from build123d import *

# Parameters (mm, degrees)
F0_W     = 8.912432854
F0_H     = 0.0079375
F0_W_2   = 2.54
F0_W_3   = 18.0631426697
F1_DEPTH = 2.1082


with BuildPart() as f1:
    # F0 (on Right) → F1 (new body)
    with BuildSketch(Plane.YZ):
        with BuildLine():
            Line((0, 162.0091375), (0, 0))
            Line((0, 0), (12.335197777, 0))
            Line((12.335197777, 0), (18.8042013144, 29.896105485))
            Line((18.8042013144, 29.896105485), (30.5493542935, 2.3257501254))
            Line((30.5493542935, 2.3257501254), (31.5401391658, 0))
            Line((31.5401391658, 0), (31.5707651968, 0))
            Line((31.5707651968, 0), (40.8442968098, 0))
            Line((40.8442968098, 0), (20.5594925834, 47.616175108))
            Line((20.5594925834, 47.616175108), (39.5771112022, 135.5049402038))
            Line((39.5771112022, 135.5049402038), (73.5248959406, 160.7899383022))
            Line((73.5248959406, 160.7899383022), (100.203, 160.7899383022))
            Line((100.203, 160.7899383022), (100.203, 162.0091375))
            Line((100.203, 162.0091375), (82.1398573303, 162.0091375))
            ThreePointArc((82.1398573303, 162.0091375), (80.3438061061, 162.7530862758), (79.5998573303, 164.5491375))
            Line((79.5998573303, 164.5491375), (79.5998573303, 169.3418))
            Line((79.5998573303, 169.3418), (70.6874244764, 169.3418))
            Line((70.6874244764, 169.3418), (70.6874244764, 165.8480664454))
            Line((70.6874244764, 165.8480664454), (70.6874244764, 164.5491375))
            ThreePointArc((70.6874244764, 164.5491375), (70.0510915867, 162.8675752701), (68.4609272063, 162.0285589874))
            ThreePointArc((68.4609272063, 162.0285589874), (68.3044763435, 162.0139975214), (68.1474244764, 162.0091375))
            Line((68.1474244764, 162.0091375), (0, 162.0091375))
        make_face()
        Polygon((21.4843682503, 35.8535070154), (23.4753466245, 31.1799211209), (21.1385536773, 30.1844319338), (19.147575303, 34.8580178283), align=None, mode=Mode.SUBTRACT)
        Polygon((25.8665425285, 25.5668719827), (27.8575209028, 20.8932860882), (25.5207279555, 19.8977969011), (23.5297495813, 24.5713827956), align=None, mode=Mode.SUBTRACT)
        with BuildLine():
            Line((12.3986134924, 50.3752630702), (11.6175919588, 46.7658196656))
            Line((11.6175919588, 46.7658196656), (10.5918, 46.7658196656))
            Line((10.5918, 46.7658196656), (10.5918, 158.7579375))
            Line((10.5918, 158.7579375), (35.8507619547, 158.7579375))
            Line((35.8507619547, 158.7579375), (31.8897708968, 140.4524587956))
            Line((31.8897708968, 140.4524587956), (31.1087493632, 136.8430153909))
            Line((31.1087493632, 136.8430153909), (35.5475592049, 135.882533211))
            ThreePointArc((35.5475592049, 135.882533211), (37.1456481821, 134.7755682604), (37.4929253116, 132.8628062845))
            Line((37.4929253116, 132.8628062845), (29.5595533377, 96.1992113407))
            ThreePointArc((29.5595533377, 96.1992113407), (28.452588387, 94.6011223635), (26.5398264112, 94.2538452339))
            Line((26.5398264112, 94.2538452339), (22.1010165695, 95.2143274138))
            Line((22.1010165695, 95.2143274138), (21.7536814278, 93.6091392306))
            Line((21.7536814278, 93.6091392306), (21.4063462861, 92.0039510473))
            Line((21.4063462861, 92.0039510473), (25.8451561277, 91.0434688674))
            ThreePointArc((25.8451561277, 91.0434688674), (27.4432451049, 89.9365039168), (27.7905222345, 88.0237419409))
            Line((27.7905222345, 88.0237419409), (19.8571502605, 51.3601469971))
            ThreePointArc((19.8571502605, 51.3601469971), (18.7501853099, 49.7620580199), (16.837423334, 49.4147808903))
            Line((16.837423334, 49.4147808903), (12.3986134924, 50.3752630702))
        make_face(mode=Mode.SUBTRACT)
        Polygon((47.0613097153, 149.2568137468), (48.5785484084, 147.2197602993), (44.5044415132, 144.1852829132), (42.9872028202, 146.2223363607), align=None, mode=Mode.SUBTRACT)
        Polygon((44.8088104432, 150.074821282), (46.6876875952, 158.7579375), (56.4668125154, 158.7579375), align=None, mode=Mode.SUBTRACT)
        Polygon((63.2751536106, 161.3332132886), (64.7923923036, 159.296159841), (60.7182854085, 156.2616824549), (59.2010467154, 158.2987359025), align=None, mode=Mode.SUBTRACT)
        with BuildLine():
            Line((0, 164.5491375), (0, 162.0091375))
            Line((0, 162.0091375), (68.1474244764, 162.0091375))
            ThreePointArc((68.1474244764, 162.0091375), (68.3044763435, 162.0139975214), (68.4609272063, 162.0285589874))
            Line((68.4609272063, 162.0285589874), (69.6856973646, 162.9407926238))
            Line((69.6856973646, 162.9407926238), (68.1474244764, 165.0060867035))
            Line((68.1474244764, 165.0060867035), (68.1474244764, 164.5491375))
            Line((68.1474244764, 164.5491375), (55.1748093832, 164.5491375))
            Line((55.1748093832, 164.5491375), (50.0948093832, 164.5491375))
            Line((50.0948093832, 164.5491375), (10.3999171089, 164.5491375))
            Line((10.3999171089, 164.5491375), (5.3199171089, 164.5491375))
            Line((5.3199171089, 164.5491375), (0, 164.5491375))
        make_face()
        Polygon((18.8042013144, 29.896105485), (12.335197777, 0), (13.2072197655, 0), (31.5401391658, 0), (30.5493542935, 2.3257501254), align=None)
        Polygon((0, 169.3418), (0, 164.5491375), (5.3199171089, 164.5491375), (5.3199171089, 167.0891375), (10.3999171089, 167.0891375), (10.3999171089, 164.5491375), (50.0948093832, 164.5491375), (50.0948093832, 167.0891375), (55.1748093832, 167.0891375), (55.1748093832, 164.5491375), (68.1474244764, 164.5491375), (68.1474244764, 165.0060867035), (68.1474244764, 169.3418), align=None)
        with BuildLine():
            Line((69.6856973646, 162.9407926238), (68.4609272063, 162.0285589874))
            ThreePointArc((68.4609272063, 162.0285589874), (70.0510915867, 162.8675752701), (70.6874244764, 164.5491375))
            Line((70.6874244764, 164.5491375), (70.6874244764, 165.8480664454))
            Line((70.6874244764, 165.8480664454), (70.6874244764, 169.3418))
            Line((70.6874244764, 169.3418), (68.1474244764, 169.3418))
            Line((68.1474244764, 169.3418), (68.1474244764, 165.0060867035))
            Line((68.1474244764, 165.0060867035), (69.6856973646, 162.9407926238))
        make_face()
        with Locations((75.1436409033, 169.34576875)):
            Rectangle(F0_W, F0_H)
        with Locations((80.8698573303, 169.34576875)):
            Rectangle(F0_W_2, F0_H)
        with BuildLine():
            Line((82.1398573303, 169.3418), (79.5998573303, 169.3418))
            Line((79.5998573303, 169.3418), (79.5998573303, 164.5491375))
            ThreePointArc((79.5998573303, 164.5491375), (80.3438061061, 162.7530862758), (82.1398573303, 162.0091375))
            Line((82.1398573303, 162.0091375), (100.203, 162.0091375))
            Line((100.203, 162.0091375), (100.203, 164.5491375))
            Line((100.203, 164.5491375), (89.6502663064, 164.5491375))
            Line((89.6502663064, 164.5491375), (84.5702663064, 164.5491375))
            Line((84.5702663064, 164.5491375), (82.1398573303, 164.5491375))
            Line((82.1398573303, 164.5491375), (82.1398573303, 169.3418))
        make_face()
        with Locations((91.1714286652, 169.34576875)):
            Rectangle(F0_W_3, F0_H)
        Polygon((100.203, 169.3418), (82.1398573303, 169.3418), (82.1398573303, 164.5491375), (84.5702663064, 164.5491375), (84.5702663064, 167.0891375), (89.6502663064, 167.0891375), (89.6502663064, 164.5491375), (100.203, 164.5491375), align=None)
        Polygon((10.5918, 46.7658196656), (11.6175919588, 46.7658196656), (12.3986134924, 50.3752630702), (12.9357939022, 52.8578095868), (20.8691658762, 89.5214045307), (21.4063462861, 92.0039510473), (21.7536814278, 93.6091392306), (22.1010165695, 95.2143274138), (22.6381969794, 97.6968739305), (30.5715689534, 134.3604688743), (31.1087493632, 136.8430153909), (31.8897708968, 140.4524587956), (35.8507619547, 158.7579375), (10.5918, 158.7579375), align=None)
        with BuildLine():
            Line((12.9357939022, 52.8578095868), (12.3986134924, 50.3752630702))
            Line((12.3986134924, 50.3752630702), (16.837423334, 49.4147808903))
            ThreePointArc((16.837423334, 49.4147808903), (18.7501853099, 49.7620580199), (19.8571502605, 51.3601469971))
            Line((19.8571502605, 51.3601469971), (27.7905222345, 88.0237419409))
            ThreePointArc((27.7905222345, 88.0237419409), (27.4432451049, 89.9365039168), (25.8451561277, 91.0434688674))
            Line((25.8451561277, 91.0434688674), (21.4063462861, 92.0039510473))
            Line((21.4063462861, 92.0039510473), (20.8691658762, 89.5214045307))
            Line((20.8691658762, 89.5214045307), (25.3079757178, 88.5609223508))
            Line((25.3079757178, 88.5609223508), (24.0175885553, 82.5974767434))
            Line((24.0175885553, 82.5974767434), (22.9432277355, 77.6323837102))
            Line((22.9432277355, 77.6323837102), (19.7419229759, 62.8377489213))
            Line((19.7419229759, 62.8377489213), (18.6675621562, 57.872655888))
            Line((18.6675621562, 57.872655888), (17.3746037439, 51.8973274069))
            Line((17.3746037439, 51.8973274069), (12.9357939022, 52.8578095868))
        make_face()
        Polygon((20.8691658762, 89.5214045307), (12.9357939022, 52.8578095868), (17.3746037439, 51.8973274069), (18.6675621562, 57.872655888), (16.1850156395, 58.4098362979), (17.2593764593, 63.3749293312), (19.7419229759, 62.8377489213), (22.9432277355, 77.6323837102), (20.4606812189, 78.16956412), (21.5350420386, 83.1346571533), (24.0175885553, 82.5974767434), (25.3079757178, 88.5609223508), align=None)
        with BuildLine():
            Line((35.5475592049, 135.882533211), (31.1087493632, 136.8430153909))
            Line((31.1087493632, 136.8430153909), (30.5715689534, 134.3604688743))
            Line((30.5715689534, 134.3604688743), (35.010378795, 133.3999866944))
            Line((35.010378795, 133.3999866944), (33.7174203827, 127.4246582133))
            Line((33.7174203827, 127.4246582133), (32.643059563, 122.45956518))
            Line((32.643059563, 122.45956518), (29.4417548033, 107.6649303911))
            Line((29.4417548033, 107.6649303911), (28.3673939836, 102.6998373579))
            Line((28.3673939836, 102.6998373579), (27.077006821, 96.7363917505))
            Line((27.077006821, 96.7363917505), (22.6381969794, 97.6968739305))
            Line((22.6381969794, 97.6968739305), (22.1010165695, 95.2143274138))
            Line((22.1010165695, 95.2143274138), (26.5398264112, 94.2538452339))
            ThreePointArc((26.5398264112, 94.2538452339), (28.452588387, 94.6011223635), (29.5595533377, 96.1992113407))
            Line((29.5595533377, 96.1992113407), (37.4929253116, 132.8628062845))
            ThreePointArc((37.4929253116, 132.8628062845), (37.1456481821, 134.7755682604), (35.5475592049, 135.882533211))
        make_face()
        Polygon((35.010378795, 133.3999866944), (30.5715689534, 134.3604688743), (22.6381969794, 97.6968739305), (27.077006821, 96.7363917505), (28.3673939836, 102.6998373579), (25.884847467, 103.2370177677), (26.9592082867, 108.202110801), (29.4417548033, 107.6649303911), (32.643059563, 122.45956518), (30.1605130463, 122.9967455899), (31.2348738661, 127.9618386231), (33.7174203827, 127.4246582133), align=None)
        Polygon((56.4668125154, 158.7579375), (46.6876875952, 158.7579375), (44.8088104432, 150.074821282), align=None)
    extrude(amount=F1_DEPTH)


solid = f1.part
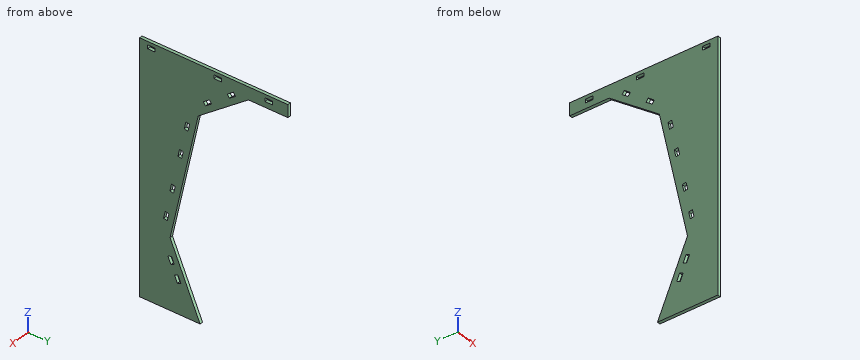
Part model, mm, in its own coordinate system. Coordinates: 2 decimals unless noted, no trailing zeros. Loops run counter-clockwise (first coordinate to the right, second up) from the corner with the lowest first, then second, coordinate; pieces in that order, holes last. Notation, with made-up numbers: (-2.5, 69) -> (23.5, 69) arc R30 cw to (23.5, 107) -> close; hole circle Ø6 at (80, 84). An arc over 180 degrees is marked (long way). Use a Markdown table: item, result. Add a question column.
Item 1: Band-saw the part on C-C on z = 11. Write the cut outline in (x, y), plus the area to 3 significant figures.
Item 2: Probe probe 1 along Z at (x, y) = (0.3, 85); probe 2 along Y at (x, z) = (0.5, 126); probe 3 along Z at (x, y) = (1, 84). List the from-to ranges inside material, lowest first.
Item 3: Band-saw the part on A-A on x = 0.55. Give the number of separate pieces and of enclosed holes in the cut face, plus the area to 3 significant figures.
Item 4: Band-saw the part on B-B on y = 76. Write the cut outline in (x, z), plus the area to 3 significant figures.
Item 5: Flat gauge pin, fed straight in: P1, Ø0.6, axis at x = 1.5, y = 87, coming from the -Z side. Where does the tip first touch, or does it go through?
Geometry says:
| question | item | result |
|---|---|---|
| 1 | outline | (0, 0) -> (2.11, 0) -> (2.11, 36.16) -> (0, 36.16) -> close |
| 1 | area | 76.2 mm² |
| 2 | probe 1 | 160.79 to 164.55, 167.09 to 169.35 |
| 2 | probe 2 | 0 to 30.81, 33.41 to 37.52 |
| 2 | probe 3 | 160.79 to 169.35 |
| 3 | separate pieces | 1 |
| 3 | enclosed holes | 11 |
| 3 | area | 6,250 mm² |
| 4 | outline | (0, 160.79) -> (2.11, 160.79) -> (2.11, 169.35) -> (0, 169.35) -> close |
| 4 | area | 18.0 mm² |
| 5 | P1 | z = 160.79 |
